Read the model definition and answer for the solid it produces. Units are mm, in the model's axes. Face numbers are marked on the shaded views. Round coordinates to 2 decimals unless told otherwise and drop trailing zeros. Loops run counter-clockwise (first coordinate to the right, second up) from the corner with the lowest first, then second, coordinate; pieces in that order, holes last. Notation, with made-up numbers: (-22, 50) -> (26, 50) arc R15 ccw to (26, 61) -> close; hole circle Ø1 at (80, -24). An arc over 180 degrees is marked (long way). Put each result on its own line as item: value.
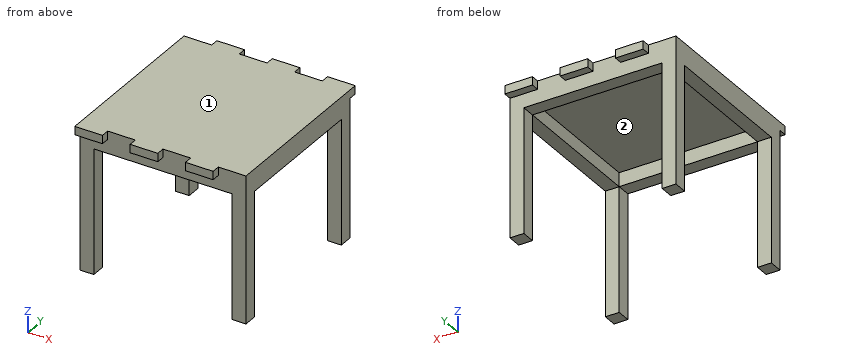
from build123d import *

# Parameters (mm, degrees)
F0_W     = 60
F0_H     = 60
F0_W_2   = 50
F0_H_2   = 50
F1_DEPTH = 5
F2_W     = 5
F2_H     = 5
F3_DEPTH = 45
F5_DEPTH = 3


with BuildPart() as f1:
    # F0 (on Top) → F1 (new body)
    with BuildSketch(Plane.XY):
        with Locations((-30, 30)):
            Rectangle(F0_W, F0_H)
        with Locations((-30, 30)):
            Rectangle(F0_W_2, F0_H_2, mode=Mode.SUBTRACT)
    extrude(amount=F1_DEPTH)

    # F2 (on face) → F3 (join)
    with BuildSketch(Plane(origin=(0, 0, 0), x_dir=(1, 0, 0), z_dir=(0, 0, -1))):
        with Locations((-2.5, -2.5)):
            Rectangle(F2_W, F2_H)
        with Locations((-57.5, -2.5)):
            Rectangle(F2_W, F2_H)
        with Locations((-2.5, -57.5)):
            Rectangle(F2_W, F2_H)
        with Locations((-57.5, -57.5)):
            Rectangle(F2_W, F2_H)
    extrude(amount=F3_DEPTH)

    # F4 (on face) → F5 (join)
    with BuildSketch(Plane.XY.offset(5)):
        Polygon((-10, 0), (0, 0), (0, 63), (-10, 63), (-10, 60), align=None)
        Polygon((-10, -3), (-10, 0), (-10, 60), (-20, 60), (-20, 0), (-20, -3), align=None)
        Polygon((-20, 0), (-20, 60), (-20, 63), (-30, 63), (-30, 60), (-30, 0), align=None)
        Polygon((-30, -3), (-30, 0), (-30, 60), (-40, 60), (-40, 0), (-40, -3), align=None)
        Polygon((-40, 0), (-40, 60), (-40, 63), (-50, 63), (-50, 60), (-50, 0), align=None)
        Polygon((-50, -3), (-50, 0), (-50, 60), (-60, 60), (-60, -3), align=None)
    extrude(amount=F5_DEPTH)


solid = f1.part
Item 1: The part is cut by section C-C (x = -26). Determine the outline of the cut face in (y, z), then the cut area to 3 significant figures.
Derived:
outline: (0, 0) -> (5, 0) -> (5, 5) -> (55, 5) -> (55, 0) -> (60, 0) -> (60, 5) -> (63, 5) -> (63, 8) -> (0, 8) -> close
area: 239 mm^2
Item 2: For a pull along Y with two mould halves and no side action, classify the marked faces 1 and 2 as pulls with the +Y half, pulls with the -Y half, needs draft (parallel to the pull), parting line crosses it, or undercut.
Derived:
face 1: needs draft
face 2: undercut
Item 3: Flat-ended cylindrical pins translate along their axes: pin 1 Ø5 at (x, z) = (-22.5, -4) entering from -Y; pin 2 Ø1.5 at (y, z) = (-1, 7) entering from +X; pin 3 Ø2.5 at (x, y) = (-33, -1) entering from -Z; pin 4 Ø6 at (y, z) = (6, -39) entering from +X. Find the tip coordinate at first contact, or state that the pin passes through.
Derived:
pin 1: passes through
pin 2: stops at x = -10
pin 3: stops at z = 0
pin 4: stops at x = 0
Item 4: Find the intervals of material crossed by line 1 along Y through (x, z) = (-3, -34); line 2 along Z through (x, y) = (-26, 18); line 3 along Z through (x, y) = (-3.5, 16), in increasing order.
Derived:
line 1: y = 0 to 5, 55 to 60
line 2: z = 5 to 8
line 3: z = 0 to 8
Item 5: The part is cut by section D-D (y = 27). Determine the outline of the cut face in (x, z), then the cut area to 3 significant figures.
Derived:
outline: (-60, 0) -> (-55, 0) -> (-55, 5) -> (-5, 5) -> (-5, 0) -> (0, 0) -> (0, 8) -> (-60, 8) -> close
area: 230 mm^2
Item 6: The part is cut by section B-B (y = 3). Determine the outline of the cut face in (x, z).
Derived:
outline: (-60, -45) -> (-55, -45) -> (-55, 0) -> (-5, 0) -> (-5, -45) -> (0, -45) -> (0, 8) -> (-60, 8) -> close
Item 7: The part is cut by section A-A (z = -26). Determine the outline of the cut face in (x, y).
Derived:
outline: (-60, 0) -> (-55, 0) -> (-55, 5) -> (-60, 5) -> close; (-60, 55) -> (-55, 55) -> (-55, 60) -> (-60, 60) -> close; (-5, 0) -> (0, 0) -> (0, 5) -> (-5, 5) -> close; (-5, 55) -> (0, 55) -> (0, 60) -> (-5, 60) -> close
